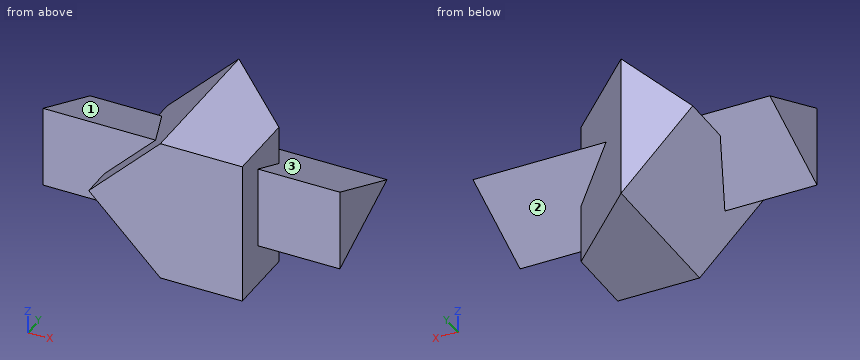
```python
from build123d import *

# Parameters (mm, degrees)
EXTRUDE1_DEPTH      = 75
CUT_EXTRUDE1_DEPTH  = 71
EXTRUDE2_DEPTH      = 40
EXTRUDE2_DEPTH_BACK = 105


with BuildPart() as part:
    # Sketch1 → Extrude1 (new body)
    with BuildSketch(Plane(origin=(0, 0, 0), x_dir=(1, 0, 0), z_dir=(0, 1, 0))):
        Polygon((0, 0), (35, 35), (75, 35), (75, -35), (35, -35), align=None)
    extrude(amount=EXTRUDE1_DEPTH)

    # Sketch2 → Cut-Extrude1 (cut, through all)
    with BuildSketch(Plane.XY.offset(35)):
        Polygon((35, 75), (75, 35), (75, 75), align=None)
    extrude(amount=-CUT_EXTRUDE1_DEPTH, mode=Mode.SUBTRACT)

    # Sketch3 → Extrude2 (add, two sides)
    with BuildSketch(Plane(origin=(75, 0, 0), x_dir=(0, 0, -1), z_dir=(1, 0, 0))) as extrude2_sk:
        Polygon((-25, 15), (15, 15), (-5, 60), align=None)
    extrude(amount=EXTRUDE2_DEPTH)
    extrude(extrude2_sk.sketch, amount=-EXTRUDE2_DEPTH_BACK)


solid = part.part
```
Design review of the part built by this model. Coordinates are the model's own, in mm. Face numbers are marked on the shaded views. A direction names the side the tool comes from. Coordinates: 2 decimals unless noted, no trailing zeros. Order: outer loops, then holes, each group sorted by start corner. A loop starts at its lowest first (then second) coordinate and runs counter-clockwise, first axis right, second up. Notation, with made-up numbers: (9, 4.5) -> (50, 4.5) arc R26 cw to (50, 36.5) -> close; hole circle Ø6 at (2, -1.75). An arc over 180 degrees is marked (long way). One line per item, written item: value. Start each with the question number.
Q1. Take a section at D-D, the plane z = 22. State the section outline as (x, y) points.
Q2. Take a section at A-A, the plane z = -4. State the section outline as (x, y) points.
Q3. Take a section at B-B, the plane x = 7. State the section outline as (y, z) points, then the cut area to 3 significant figures.
Q4. Tool access review of the marked faces 1, 2 and 3: name each direction out of +Z, -Z, +X, -X, +Y, -Y from which nothing blocks a thin tool from reaching the whole face with its end or side.
Q5. Take a section at C-C, the plane y = 24. State the section outline as (x, z) points, then the cut area to 3 significant figures.
Q6. Insertion check: pin 1 Ø1.5 at (x, y) = (15, 17.5) entering from -Z; pin 2 Ø8 at (y, z) = (47, 24.5) entering from -X; pin 3 Ø2 at (x, y) = (99, 21) entering from +Z. Each pin has a flat end and moves straight along its axis. Give the tip position at first contact, or say it passes through.
Q7. For probe 1 along Z at (x, y) = (32, 44); probe 2 along Y at (x, z) = (8.5, 13); probe 3 along X at (y, z) = (39, -13), list the stretches that pass through material, from the lowest coordinate up.
Values follow:
1. outline: (-30, 15) -> (22, 15) -> (22, 0) -> (75, 0) -> (75, 15) -> (115, 15) -> (115, 21.75) -> (75, 21.75) -> (75, 35) -> (35, 75) -> (22, 75) -> (22, 21.75) -> (-30, 21.75) -> close
2. outline: (-30, 15) -> (4, 15) -> (4, 0) -> (75, 0) -> (75, 15) -> (115, 15) -> (115, 39.75) -> (70.25, 39.75) -> (35, 75) -> (4, 75) -> (4, 39.75) -> (-30, 39.75) -> close
3. outline: (0, -7) -> (15, -7) -> (15, -15) -> (33, -7) -> (75, -7) -> (75, 7) -> (55.5, 7) -> (15, 25) -> (15, 7) -> (0, 7) -> close
3. area: 1,490 mm2
4. face 1: +Z, -X, +Y
4. face 2: -Z, +X, +Y
4. face 3: +Z, +X, +Y
5. outline: (-30, -11) -> (11, -11) -> (35, -35) -> (75, -35) -> (75, -11) -> (115, -11) -> (115, 21) -> (75, 21) -> (75, 35) -> (35, 35) -> (21, 21) -> (-30, 21) -> close
5. area: 6,550 mm2
6. pin 1: stops at z = -15.75
6. pin 2: stops at x = 20.5
6. pin 3: stops at z = 22.78
7. probe 1: z = -32 to 32
7. probe 2: y = 15 to 42
7. probe 3: x = 13 to 71
